from build123d import *

# Parameters (mm, degrees)
F0_W     = 228.6
F0_H     = 101.6
F1_DEPTH = 304.8
F2_T     = -6.35
F3_W     = 58.928
F3_H     = 86.868
F4_DEPTH = 25.4


with BuildPart() as f1:
    # F0 (on Top) → F1 (new body)
    with BuildSketch(Plane.XY):
        Rectangle(F0_W, F0_H)
    extrude(amount=F1_DEPTH)

    # F2
    f2_openings = [f1.faces().sort_by_distance(p)[0] for p in [
        (0, 50.8, 152.4),
    ]]
    offset(amount=F2_T, openings=f2_openings)

    # F3 (on face) → F4 (cut)
    with BuildSketch(Plane.XZ.offset(50.8)):
        with Locations((53.086, 229.616)):
            Rectangle(F3_W, F3_H)
        with Locations((53.086, 110.998)):
            Rectangle(F3_W, F3_H)
    extrude(amount=-F4_DEPTH, mode=Mode.SUBTRACT)


solid = f1.part
Input: part model. Units: mm. Frame: model coordinates. A direction names the side the tool comes from. Coordinates: 2 decimals unless noted, no trailing zeros. Order: outer loops, then holes, each group sorted by start corner. A loop starts at its lowest first (then second) coordinate and runs counter-clockwise, first axis right, second up. Notation, with made-up numbers: M 75.25,1.25 L 121.25,1.25 A19 ccw 121.25,35.25 Z; hole C 32.5,-3.5 d10. An arc over 180 degrees is marked long. Write item = value, one per line. Start each with the question number.
(1) Reachability of faces 1 (the flat face through (-2, 4, 6.35)), 2 (the flat face through (53, -48, 186.182)), 3 (the flat face through (-2, 1, 304.8)) from +Z, -Z, +X, -X, +Y, -Y: full face, straight path, thin tool, end or side. Return the list, or none.
(2) Line query: line 1 along X through (y, z) = (-3, 29.5); line 2 along Z through (x, y) = (-5.5, 42.5); line 3 along Y through (x, z) = (-89.5, 171.5). Output: solid intervals per line, ascending. Write a range as [from, to].
(3) Section D-D on z = 281.5. Output: boundary loops of the cut face in (x, y).
(4) Section B-B on y = -4.5. Output: boundary loops of the cut face in (x, z), and give its area (3 significant figures).
(5) Section A-A on z = 106.5. Output: boundary loops of the cut face in (x, y), and give its area (3 significant figures).
(6) Section C-C on x = 94. Output: boundary loops of the cut face in (y, z), and give its area (3 significant figures).
(7) First-contact query: P1, Ø1.5, axis at x = 81, z = 234.5, coming from the +Y side; P2, Ø1, axis at x = -41.5, z = 158, coming from the +Y side. Flat tips, straight axial feed; report the tip coordinate or a pass-through.
Result set:
q1.face_1 = +Y
q1.face_2 = +Y, -Y
q1.face_3 = +Z, +X, -X, +Y, -Y
q2.line_1 = [-114.3, -107.95], [107.95, 114.3]
q2.line_2 = [0, 6.35], [298.45, 304.8]
q2.line_3 = [-50.8, -44.45]
q3.outline = M -114.3,-50.8 L 114.3,-50.8 L 114.3,50.8 L 107.95,50.8 L 107.95,-44.45 L -107.95,-44.45 L -107.95,50.8 L -114.3,50.8 Z
q4.outline = M -114.3,0 L 114.3,0 L 114.3,304.8 L -114.3,304.8 Z; hole M -107.95,6.35 L 107.95,6.35 L 107.95,298.45 L -107.95,298.45 Z
q4.area = 6,610 mm²
q5.outline = M -114.3,-50.8 L 23.62,-50.8 L 23.62,-44.45 L -107.95,-44.45 L -107.95,50.8 L -114.3,50.8 Z; M 82.55,-50.8 L 114.3,-50.8 L 114.3,50.8 L 107.95,50.8 L 107.95,-44.45 L 82.55,-44.45 Z
q5.area = 2,290 mm²
q6.outline = M -50.8,0 L 50.8,0 L 50.8,6.35 L -44.45,6.35 L -44.45,298.45 L 50.8,298.45 L 50.8,304.8 L -50.8,304.8 Z
q6.area = 3,150 mm²
q7.P1 = through
q7.P2 = -44.45
